The drawing under review shows one solid part. Ordinate dimensions are in mm from its lowest x, y, z. A direction names the side the tool comes from. Give positions to 0.01 mm unless a question says otherwise; leave off trailing zeros. Order: outer loops, then holes, each group sorted by start corner. A loop starts at its lowest first (then second) coordinate and runs counter-clockwise, first axis right, second up. Notation, with made-up numbers: (57, 4.5) -> (103, 4.5) arc R21 cw to (103, 31.5) -> close; hole circle Ø10 at (16.25, -4). An arc over 180 degrees is marked (long way). One line per item, written item: value. Start each with the question number.
1) Tool access review of the marked faces 1 and 2: name each direction out of +Z, -Z, +X, -X, +Y, -Y from which nothing blocks a thin tool from reaching the whole face with its end or side.
2) Consider section A-A (x = 32.5). State the section outline as (y, z) points.
3) Wall thickness on line 1 along X through (y, z) = (15, 7.75); line 2 along X through (y, z) = (6, 0.75); line 3 along Y through (x, z) = (72, 3.5) (1 decimal): over which ranges is each line inside the solid? List them lowest first. Write a range as from..to.
4) For pin 1 (2 mm diameter, centred on x = 9, y = 8, fed in from +Z); pin 2 (1 mm diameter, centred on x = 54.5, z = 4.5, fed in from +Y); pin 3 (2 mm diameter, centred on x = 22.5, z = 9.5, fed in from -Y), all flat-tipped, find the tip position at first contact; note any pin that passes through.
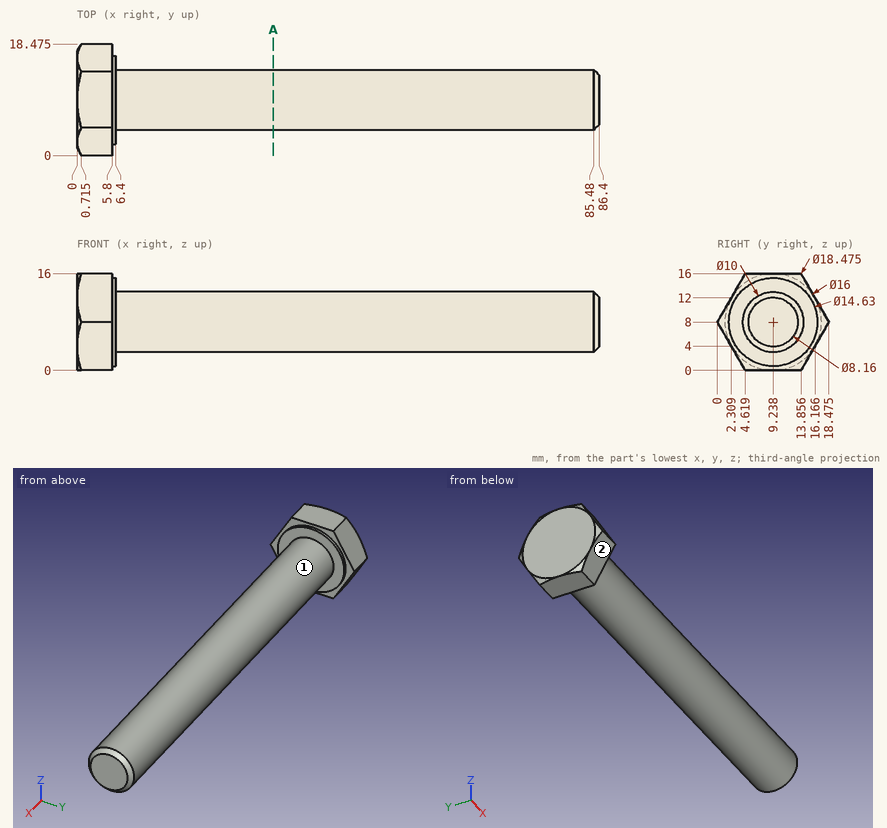
Checked values:
1. face 1: +X
1. face 2: -Z, +X, -X, -Y
2. outline: circle Ø10 at (9.24, 8)
3. line 1: x = 0..6.4
3. line 2: x = 0..5.8
3. line 3: y = 7.1..11.4
4. pin 1: stops at z = 12.99
4. pin 2: stops at y = 13.24
4. pin 3: stops at y = 4.26
